```python
from build123d import *

# Parameters (mm, degrees)
F1_DEPTH = 20
F2_W     = 19.0279083326
F2_H     = 47.3126359284
F3_DEPTH = 20
F4_W     = 19.0279083326
F4_H     = 17.7422408015
F5_DEPTH = 35
F6_W     = 19.0279087983
F6_H     = 38.1843838841
F6_H_2   = 17.7422408015
F7_DEPTH = 10


# Not quite as in the source:
# - ends of sketch curves that miss each other by under 0.0002 mm in the source are joined


with BuildPart() as f1:
    # F0 (on Front) → F1 (new body)
    with BuildSketch(Plane.XZ):
        Polygon((-6.3491990761, 71.7460297603), (-25.3968193009, 71.7460297603), (-46.6666553218, 3.8095274944), (-62.2222101619, 3.8095274944), (-62.2222101619, 0), (-38.4126887615, 0), (-38.4126887615, 3.8095274944), (-25.3968193009, 44.7619079595), (-25.3968193009, 0), (0, 0), (25.3968193009, 0), (25.3968193009, 44.7619079595), (38.4126887615, 3.8095274944), (38.4126887615, 0), (62.2222101619, 0), (62.2222101619, 3.8095274944), (46.6666553218, 3.8095274944), (25.3968193009, 71.7460297603), (6.3491990761, 71.7460297603), (6.3491990761, 76.8254005194), (11.4285635112, 76.8254005194), (11.4285635112, 100), (0, 100), (-11.4285635112, 100), (-11.4285635112, 76.8254005194), (-6.3491990761, 76.8254005194), align=None)
    extrude(amount=F1_DEPTH)

    # F2 (on Top) → F3 (join)
    with BuildSketch(Plane.XY):
        with Locations((-16.1994355731, 23.6563179642)):
            Rectangle(F2_W, F2_H)
        with Locations((16.1994355731, 23.6563179642)):
            Rectangle(F2_W, F2_H)
    extrude(amount=F3_DEPTH)

    # F4 (on Top) → F5 (join)
    with BuildSketch(Plane.XY):
        with Locations((16.1994318478, 38.6986536905)):
            Rectangle(F4_W, F4_H)
        with Locations((-16.1994318478, 38.6986536905)):
            Rectangle(F4_W, F4_H)
    extrude(amount=-F5_DEPTH)

    # F6 (on face) → F7 (join)
    with BuildSketch(Plane(origin=(0, 0, -35), x_dir=(1, 0, 0), z_dir=(0, 0, -1))):
        Polygon((25.7133860141, -68.0119171739), (25.7133860141, -47.5697740912), (6.6854776815, -47.5697740912), (6.6854772158, -68.0119171739), align=None)
        with Locations((-16.199431615, -48.9197252318)):
            Rectangle(F6_W, F6_H)
        with Locations((16.199431615, -38.6986536905)):
            Rectangle(F6_W, F6_H_2)
    extrude(amount=F7_DEPTH)


solid = f1.part
```
The model under review builds one solid part; all positions refer to its coordinate system, in mm. A direction names the side the tool comes from. Round coordinates to 2 decimals unless told otherwise and drop trailing zeros. Loops run counter-clockwise (first coordinate to the right, second up) from the corner with the lowest first, then second, coordinate; pieces in that order, holes last. Notation, with made-up numbers: (55, 13) -> (59, 13) arc R11 cw to (59, 29) -> close; hole circle Ø1 at (53, -11). An arc over 180 degrees is marked (long way). Answer as a JSON object with one key per item and string values. Group by question number.
1) For pin 1 Ø6 at (y, z) = (-14, 93) entering from -X; pin 2 Ø5 at (y, z) = (60.5, -40) entering from -X; pin 3 Ø1.5 at (x, y) = (9.5, -11.5) entering from -Z, all flat-tipped, find the tip position at first contact; note any pin that passes through.
2) We need section D-D on y = -13. Write out the cut boundary in (x, z).
3) We need section A-A on z = -30. Write out the cut boundary in (x, y), then the cut area to 3 significant figures.
4) We need section C-C on x = 9. Write out the cut boundary in (y, z), then the cut area to 3 significant figures.
5) For faces 1 (the face through (-16, 24, 20)), 2 (the face through (16, 29.828, -22)), 3 (the face through (-6.685, 23, 10)), 4 (the face through (6.349, -10, 74)), 5 (the face through (38.413, -10, 2)), list the 3-axis set-ups (+Z, -Z, +X, -X, +Y, -Y) from which the entire face can be reached by the end or side of a thin tool; tool diameter is ignored.
6) Mouldability with a two-part tool opening along Z and no side actions: class faces 6 (the face through (50, -10, 0)), 7 (the face through (-25.713, 23, 10)), 8 (the face through (-9, -10, 76.825)) as released by +Z, released by -Z, zero draft, split by the parting line, or undercut.
7) For line 1 (X direction, y = -1.5, z = 2); line 2 (X direction, y = 41, z = -18); line 3 (Z direction, x = 9, y = -1), list the stretches that pass through material, from the lowest coordinate up. Write a range as [from, to].
Result set:
{
 "1": {"pin 1": "x = -11.43", "pin 2": "x = -25.71", "pin 3": "z = 0"},
 "2": {"outline": "(-62.22, 0) -> (-38.41, 0) -> (-38.41, 3.81) -> (-25.4, 44.76) -> (-25.4, 0) -> (25.4, 0) -> (25.4, 44.76) -> (38.41, 3.81) -> (38.41, 0) -> (62.22, 0) -> (62.22, 3.81) -> (46.67, 3.81) -> (25.4, 71.75) -> (6.35, 71.75) -> (6.35, 76.83) -> (11.43, 76.83) -> (11.43, 100) -> (-11.43, 100) -> (-11.43, 76.83) -> (-6.35, 76.83) -> (-6.35, 71.75) -> (-25.4, 71.75) -> (-46.67, 3.81) -> (-62.22, 3.81) -> close"},
 "3": {"outline": "(-25.71, 29.83) -> (-6.69, 29.83) -> (-6.69, 47.57) -> (-25.71, 47.57) -> close; (6.69, 29.83) -> (25.71, 29.83) -> (25.71, 47.57) -> (6.69, 47.57) -> close", "area": "675 mm²"},
 "4": {"outline": "(-20, 0) -> (29.83, 0) -> (29.83, -45) -> (68.01, -45) -> (68.01, -35) -> (47.57, -35) -> (47.57, 0) -> (47.31, 0) -> (47.31, 20) -> (0, 20) -> (0, 71.75) -> (-20, 71.75) -> close; (-20, 76.83) -> (0, 76.83) -> (0, 100) -> (-20, 100) -> close", "area": "3,850 mm²"},
 "5": {"face 1": "+Z, +X, -X, +Y", "face 2": "-Z, +X, -X, -Y", "face 3": "+Z, -Z, +Y", "face 4": "+X, +Y, -Y", "face 5": "-Z, +Y, -Y"},
 "6": {"face 6": "released by -Z", "face 7": "zero draft", "face 8": "undercut"},
 "7": {"line 1": "[-62.22, -38.41], [-25.4, 25.4], [38.41, 62.22]", "line 2": "[-25.71, -6.69], [6.69, 25.71]", "line 3": "[0, 71.75], [76.83, 100]"}
}
